Autodesk Inventor part; units mm, degrees
ref_plane "YZ Plane" through (0, 0, 0) normal (1, 0, 0) x (0, 1, 0)
ref_plane "XZ Plane" through (0, 0, 0) normal (0, 1, 0) x (-1, 0, 0)
ref_plane "XY Plane" through (0, 0, 0) normal (0, 0, 1) x (1, 0, 0)
sketch "Эскиз1" plane through (0, 0, 0) normal (0, 0, 1) x (1, 0, 0)
  line L0 (-42, -20) -> (42, -20)
  line L1 (42, -20) -> (42, 20)
  line L2 (42, 20) -> (-42, 20)
  line L3 (-42, 20) -> (-42, -20)
  line L4 (-42, -20) -> (42, 20) construction
  line L5 (42, -20) -> (-42, 20) construction
  line L6 (-42, 20) -> (-40, 20)
  line L7 (-40, 20) -> (-40, 15)
  line L8 (-40, 15) -> (-42, 15)
  line L9 (-42, 15) -> (-42, 20)
  line L10 (42, 20) -> (35, 20)
  line L11 (35, 20) -> (35, 15)
  line L12 (35, 15) -> (42, 15)
  line L13 (42, 15) -> (42, 20)
  point P0 (0, 0)
  dimension "d0" = 84
  dimension "d1" = 40
  dimension "d3" = 5
  dimension "d4" = 2
  dimension "d20" = 75
extrude "Выдавливание1" add sketch "Эскиз1" along normal blind 1 contours L3 L8 L7 L2 L11 L12 L1 L0
sketch "Эскиз2" plane through (0, 0, 0) normal (0, 0, -1) x (-1, 0, 0)
  line L0 (40, 8.5) -> (-35, 8.5)
  line L1 (-35, 8.5) -> (-35, 23.5)
  line L2 (-35, 23.5) -> (40, 23.5)
  line L3 (40, 23.5) -> (40, 8.5)
  line L4 (-35, 20) -> (40, 20)
  point P0 (0, 0)
  point P1 (40, 15)
  point P2 (-35, 15)
  dimension "d7" = 3.5
  dimension "d8" = 15
extrude "Выдавливание2" add sketch "Эскиз2" along normal blind 13.5
sketch "Эскиз3" plane through (0, 0, 1) normal (0, 0, 1) x (1, 0, 0)
  circle A0 centre (4, -17) radius 1
  line L0 (-42, -20) -> (42, -20)
  line L1 (-42, 15) -> (-42, -20)
  circle A1 centre (38, 0) radius 1
  line L2 (42, 15) -> (35, 15)
  line L3 (42, -20) -> (42, 15)
  point P0 (0, 0)
  dimension "d11" = 2
  dimension "d12" = 3
  dimension "d13" = 46
  dimension "d14" = 2
  dimension "d15" = 15
  dimension "d16" = 4
extrude "Выдавливание3" cut sketch "Эскиз3" against normal through all
sketch "Эскиз4" plane through (0, 0, 1) normal (0, 0, 1) x (1, 0, 0)
  circle A0 centre (38, 0) radius 1
  circle A1 centre (4, -17) radius 1
  line L0 (42, -20) -> (42, 15)
  line L1 (42, 15) -> (35, 15)
  line L2 (35, 15) -> (35, 20)
  line L3 (35, 20) -> (-40, 20)
  line L4 (-40, 20) -> (-40, 15)
  line L5 (-40, 15) -> (-42, 15)
  line L6 (-42, 15) -> (-42, -20)
  line L7 (-42, -20) -> (42, -20)
  line L8 (42, 15) -> (35, 15)
  line L9 (-40, 15) -> (35, 15)
  point P0 (0, 0)
properties part number "TL-SF1005D_pcb"
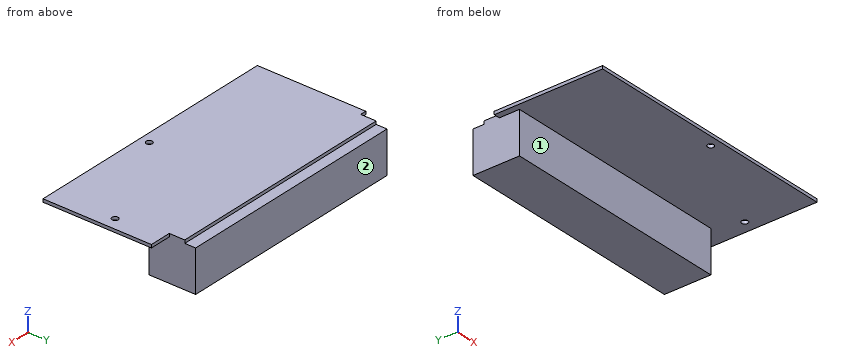
Here's how the part is built. I have some questions about the finished solid (model axes, mm). Face numbers are marked on the shaded views. A direction names the side the tool comes from. Round coordinates to 2 decimals unless told otherwise and drop trailing zeros. Order: outer loops, then holes, each group sorted by start corner. A loop starts at its lowest first (then second) coordinate and runs counter-clockwise, first axis right, second up. Notation, with made-up numbers: M 52,-22 L 82,-22 A35 cw 82,11 Z; hole C 83.25,-17.5 d6. An arc over 180 degrees is marked long. One line per question, with ' | ' between items.
1) Imagine slicing it at A-A, the plane x = 38. Write out the boundary of the cut face in (y, z).
Checked values:
outline: M -20,0 L -1,0 L -1,1 L -20,1 Z; M 1,0 L 15,0 L 15,1 L 1,1 Z
2) On a 3-axis mill with a long thin cutter (end or side, diameter ignored), from which of +Z, -Z, +X, -X, +Y, -Y can I reach the whole of each face in a straight line? I mean the marked faces 1 and 2. Say none if no direction works.
Checked values:
face 1: -Z, +X, -X, -Y | face 2: +Z, -Z, +X, -X, +Y
3) I'm going to push flat-ended pins straight in: pin 1 Ø4.5 at (y, z) = (15, -4.5) entering from -X; pin 2 Ø0.5 at (x, z) = (-40.5, 0.5) entering from +Y. Where does each tip first touch, or does it pass through?
Checked values:
pin 1: stops at x = -40 | pin 2: stops at y = 15
4) I need wall thicknesses on line 1 (Y direction, x = 38, z = 0.2); line 2 (Y direction, x = 4, z = 0.5); line 3 (Z direction, x = -12, y = 1). Which ranges of each line are inside material? Lowest first, please.
Checked values:
line 1: y = -20 to -1, 1 to 15 | line 2: y = -20 to -18, -16 to 20 | line 3: z = 0 to 1
5) Imagine slicing it at B-B, the plane y = 0. Write out the boundary of the cut face in (x, z).
Checked values:
outline: M -42,0 L 37,0 L 37,1 L -42,1 Z; M 39,0 L 42,0 L 42,1 L 39,1 Z
6) Imagine slicing it at C-C, the plane x = 4. Write out the boundary of the cut face in (y, z), plus the area to 4 significant figures.
Checked values:
outline: M -20,0 L -18,0 L -18,1 L -20,1 Z; M -16,0 L 8.5,0 L 8.5,-13.5 L 23.5,-13.5 L 23.5,0 L 20,0 L 20,1 L -16,1 Z | area: 240.5 mm²
7) Imagine slicing it at D-D, the plane z = -7.5. Write out the boundary of the cut face in (x, y), plus the area to 4 significant figures.
Checked values:
outline: M -40,8.5 L 35,8.5 L 35,23.5 L -40,23.5 Z | area: 1,125 mm²
